Input: part model. Units: mm. Frame: model coordinates. Face numbers are marked on the shaded views. A direction names the side the tool comes from. Coordinates: 2 decimals unless noted, no trailing zeros. Order: outer loops, then holes, each group sorted by start corner. A loop starts at its lowest first (then second) coordinate and runs counter-clockwise, first axis right, second up. Notation, with made-up numbers: (-29, -30.5) -> (-7, -30.5) arc R20 cw to (-7, -25.5) -> close; hole circle Ø4 at (-37, 63.25). An arc over 180 degrees is marked (long way). One line per item, written item: value. Start each with the question number.
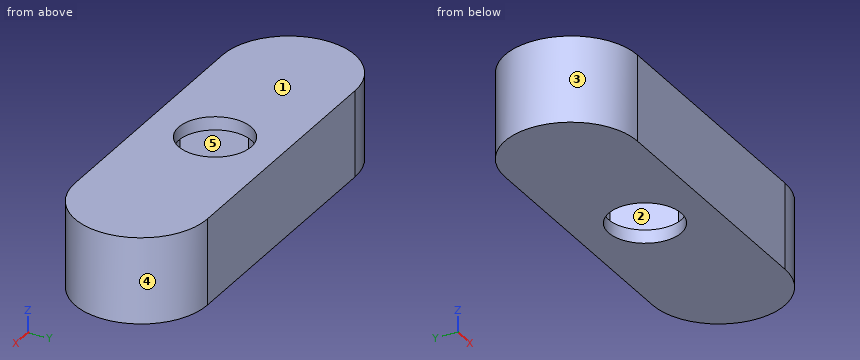
Autodesk Fusion 360 part; units mm, degrees
sketch "Sketch2" plane through (0, 0, 0) normal (0, 0, 1) x (1, 0, 0)
  line L0 (-4.5, 0) -> (4.5, 0)
  line L1 (-4.5, 0) -> (-2.25, 3.8971)
  line L2 (4.5, 0) -> (2.25, 3.8971)
  line L3 (4.5, 0) -> (9, 0) construction
  line L4 (-2.25, 3.8971) -> (2.25, 3.8971)
  line L5 (-4.5, 0) -> (-2.25, -3.8971)
  line L6 (4.5, 0) -> (2.25, -3.8971)
  line L7 (2.25, -3.8971) -> (-2.25, -3.8971)
  line L8 (-10, 5) -> (10, 5)
  line L9 (10, -5) -> (-10, -5)
  arc A0 (-10, 5) -> (-10, -5) centre (-10, 0) ccw
  arc A1 (10, -5) -> (10, 5) centre (10, 0) ccw
  circle A2 centre (0, 0) radius 2.75
  dimension "d15" = 120
  dimension "d16" = 120
  dimension "d17" = 5.5
extrude "Extrude3" add sketch "Sketch2" along normal blind 6.5 contours L0 L1 L2 L4 A2 | L0 L5 L6 L7 A2 | L8 L9 A0 A1
extrude "Extrude4" cut sketch "Sketch2" along normal blind 5.5 contours L0 L1 L2 L4 A2 | L0 L5 L6 L7 A2
extrude "Extrude5" add sketch "Sketch2" along normal blind 1 contours L0 L1 L2 L4 A2 | L0 L5 L6 L7 A2
1) Section query B-B, the plane z = 4.5. Return the cut outline in (x, y).
2) Access query for the marked faces 4 and 5. Directions: +Z, -Z, +X, -X, +Y, -Y. A direction counts if a zero-diameter tool reaches every point of the face in a straight line with its end or side. Return the directions, or none.
3) Pin query (flat end, axial travel): pin 1 Ø1.5 at (y, z) = (-2.5, 4.5) entering from +X. Return the tip coordinate at first contact, or that it passes through.
4) Section query A-A, the plane x = 0. Return the cut outline in (y, z), plus the area to 3 significant figures.
5) Section query D-D, the plane y = 3.25. Return the cut outline in (x, z).
6) Mould query, pull axis Y, two halves, no side actions, for the marked faces 1, 2 and 3. Classes: +Y half, -Y half, draft (parallel to the pull), parting line (faces both ways), or undercut.
7) Ray query, line 1 along Y through (x, z) = (0, 0.6); line 2 along X through (y, z) = (0, 0.8); line 3 along Z through (x, y) = (1.5, 3.5). Return the intervals inside material, ascending. Write a range as from..to.
8) Section query C-C, the plane y = -0.5. Return the cut outline in (x, z).
Entries:
1. outline: (-10, -5) -> (10, -5) arc R5 ccw to (10, 5) -> (-10, 5) arc R5 ccw to start; hole (-4.5, 0) -> (-2.25, -3.9) -> (2.25, -3.9) -> (4.5, 0) -> (2.25, 3.9) -> (-2.25, 3.9) -> close
2. face 4: +Z, -Z, +X
2. face 5: none
3. pin 1: stops at x = 14.68
4. outline: (-5, 0) -> (-2.75, 0) -> (-2.75, 1) -> (-3.9, 1) -> (-3.9, 5.5) -> (-2.75, 5.5) -> (-2.75, 6.5) -> (-5, 6.5) -> close; (2.75, 0) -> (5, 0) -> (5, 6.5) -> (2.75, 6.5) -> (2.75, 5.5) -> (3.9, 5.5) -> (3.9, 1) -> (2.75, 1) -> close
4. area: 18.9 mm2
5. outline: (-13.8, 0) -> (13.8, 0) -> (13.8, 6.5) -> (-13.8, 6.5) -> close; hole (-2.62, 1) -> (2.62, 1) -> (2.62, 5.5) -> (-2.62, 5.5) -> close
6. face 1: draft
6. face 2: undercut
6. face 3: parting line
7. line 1: y = -5..-2.75, 2.75..5
7. line 2: x = -15..-2.75, 2.75..15
7. line 3: z = 0..1, 5.5..6.5
8. outline: (-14.97, 0) -> (-2.7, 0) -> (-2.7, 1) -> (-4.21, 1) -> (-4.21, 5.5) -> (-2.7, 5.5) -> (-2.7, 6.5) -> (-14.97, 6.5) -> close; (2.7, 0) -> (14.97, 0) -> (14.97, 6.5) -> (2.7, 6.5) -> (2.7, 5.5) -> (4.21, 5.5) -> (4.21, 1) -> (2.7, 1) -> close
